```python
from build123d import *

# Parameters (mm, degrees)
SKETCH1_R           = 6.25
BOSS_EXTRUDE1_DEPTH = 20
BOSS_EXTRUDE2_DEPTH = 90
SKETCH3_R           = 1.75
CUT_EXTRUDE1_DEPTH  = 109.72585939
FILLET1_R           = 3
FILLET2_R           = 5


with BuildPart() as part:
    # Sketch1 → Boss-Extrude1 (new body)
    with BuildSketch(Plane(origin=(0, 0, 0), x_dir=(1, 0, 0), z_dir=(0, 1, 0))):
        with BuildLine():
            Line((0, 9.75), (11.25, 9.75))
            ThreePointArc((11.25, 9.75), (14.785533906, 8.285533906), (16.25, 4.75))
            Line((16.25, 4.75), (16.25, -9.75))
            Line((16.25, -9.75), (0, -9.75))
            ThreePointArc((0, -9.75), (-9.75, 0), (0, 9.75))
        make_face()
        with Locations(Location((0, 0, 0), (0, 0, 270))):
            Circle(SKETCH1_R, mode=Mode.SUBTRACT)
    extrude(amount=BOSS_EXTRUDE1_DEPTH)

    # Sketch2 → Boss-Extrude2 (add)
    with BuildSketch(Plane(origin=(16.25, 0, 0), x_dir=(0, 0, -1), z_dir=(1, 0, 0))):
        with BuildLine():
            Line((-6.75, 6), (-4.75, 6))
            ThreePointArc((-4.75, 6), (-2.628679656, 6.878679656), (-1.75, 9))
            Line((-1.75, 9), (-1.75, 11))
            ThreePointArc((-1.75, 11), (-2.628679656, 13.121320344), (-4.75, 14))
            Line((-4.75, 14), (-6.75, 14))
            ThreePointArc((-6.75, 14), (-8.871320344, 13.121320344), (-9.75, 11))
            Line((-9.75, 11), (-9.75, 9))
            ThreePointArc((-9.75, 9), (-8.871320344, 6.878679656), (-6.75, 6))
        make_face()
    extrude(amount=BOSS_EXTRUDE2_DEPTH)

    # Sketch3 → Cut-Extrude1 (cut, through all)
    with BuildSketch(Plane(origin=(0, 0, 1.75), x_dir=(-1, 0, 0), z_dir=(0, 0, -1))):
        with Locations(Location((-101.25, 10, 0), (0, 0, 34.849904579))):
            Circle(SKETCH3_R)
        with Locations(Location((-96.25, 10, 0), (0, 0, 34.849904579))):
            Circle(SKETCH3_R)
        with Locations(Location((-91.25, 10, 0), (0, 0, 34.849904579))):
            Circle(SKETCH3_R)
        with Locations(Location((-86.25, 10, 0), (0, 0, 34.849904579))):
            Circle(SKETCH3_R)
        with Locations(Location((-81.25, 10, 0), (0, 0, 34.849904579))):
            Circle(SKETCH3_R)
    extrude(amount=-CUT_EXTRUDE1_DEPTH, mode=Mode.SUBTRACT)

    # Fillet1
    fillet1_edges = [part.edges().sort_by_distance(p)[0] for p in [
        (106.25, 6.878679656, 8.871320344),
        (106.25, 6, 5.75),
        (106.25, 6.878679656, 2.628679656),
        (106.25, 10, 1.75),
        (106.25, 13.121320344, 2.628679656),
        (106.25, 14, 5.75),
        (106.25, 13.121320344, 8.871320344),
        (106.25, 10, 9.75),
    ]]
    fillet(fillet1_edges, radius=FILLET1_R)

    # Fillet2
    # the kernel refuses this fillet: 5 mm, written as the material it adds along each edge
    with BuildSketch(Plane(origin=(16.25, 9, 6.75), x_dir=(1.1842378929335002e-15, -0.8556201630305047, -0.5176042277799251), z_dir=(0, -0.5176042277799251, 0.8556201630305047))) as fillet2_piece_1_section:
        with BuildLine():
            CenterArc((-3 - FILLET2_R, FILLET2_R), FILLET2_R, 270, 90)
            Line((-3, FILLET2_R), (-3, 0))
            Line((-3, 0), (-3 - FILLET2_R, 0))
        make_face()
    fillet2_piece_1 = revolve(axis=Axis((16.25, 9, 6.75), (1, 0, 0)), revolution_arc=328.828315396, mode=Mode.PRIVATE)
    fillet2_piece_1 = split(fillet2_piece_1, bisect_by=Plane(origin=(16.92449451, 12.664519723, 9.75), z_dir=(0, 0, -1)), keep=Keep.TOP, mode=Mode.PRIVATE)
    add(fillet2_piece_1)
    with BuildSketch(Plane(origin=(16.25, 6, 6.75), x_dir=(0, -1, 0), z_dir=(0, 0, -1)), Plane(origin=(16.25, 9, 1.75), x_dir=(0, 0, -1), z_dir=(0, 1, 0))) as fillet2_piece_2:
        with BuildLine():
            CenterArc((FILLET2_R, -FILLET2_R), FILLET2_R, 90, 90)
            Line((0, -FILLET2_R), (0, 0))
            Line((0, 0), (FILLET2_R, 0))
        make_face()
    extrude(amount=2)
    with BuildSketch(Plane(origin=(16.25, 9, 4.75), x_dir=(0, -1, 0), z_dir=(0, 0, 1))) as fillet2_piece_3:
        with BuildLine():
            CenterArc((3 + FILLET2_R, FILLET2_R), FILLET2_R, 180, 90)
            Line((3, FILLET2_R), (3, 0))
            Line((3, 0), (3 + FILLET2_R, 0))
        make_face()
    revolve(axis=Axis((16.25, 9, 4.75), (1, 0, 0)), revolution_arc=90)
    with BuildSketch(Plane(origin=(16.25, 11, 4.75), x_dir=(0, 0, -1), z_dir=(0, -1, 0))) as fillet2_piece_4:
        with BuildLine():
            CenterArc((3 + FILLET2_R, FILLET2_R), FILLET2_R, 180, 90)
            Line((3, FILLET2_R), (3, 0))
            Line((3, 0), (3 + FILLET2_R, 0))
        make_face()
    revolve(axis=Axis((16.25, 11, 4.75), (1, 0, 0)), revolution_arc=90)
    with BuildSketch(Plane(origin=(16.25, 14, 4.75), x_dir=(1, 0, 0), z_dir=(0, 0, 1))) as fillet2_piece_5:
        with BuildLine():
            CenterArc((FILLET2_R, FILLET2_R), FILLET2_R, 180, 90)
            Line((0, FILLET2_R), (0, 0))
            Line((0, 0), (FILLET2_R, 0))
        make_face()
    extrude(amount=2)
    with BuildSketch(Plane(origin=(16.25, 11, 6.75), x_dir=(0, 1, 0), z_dir=(0, 0, -1))) as fillet2_piece_6_section:
        with BuildLine():
            CenterArc((3 + FILLET2_R, FILLET2_R), FILLET2_R, 180, 90)
            Line((3 + FILLET2_R, 0), (3, 0))
            Line((3, 0), (3, FILLET2_R))
        make_face()
    fillet2_piece_6 = revolve(axis=Axis((16.25, 11, 6.75), (1, 0, 0)), revolution_arc=328.828315396, mode=Mode.PRIVATE)
    fillet2_piece_6 = split(fillet2_piece_6, bisect_by=Plane(origin=(17.971658099, 13.274254424, 9.75), z_dir=(0, 0, -1)), keep=Keep.TOP, mode=Mode.PRIVATE)
    add(fillet2_piece_6)


solid = part.part
```
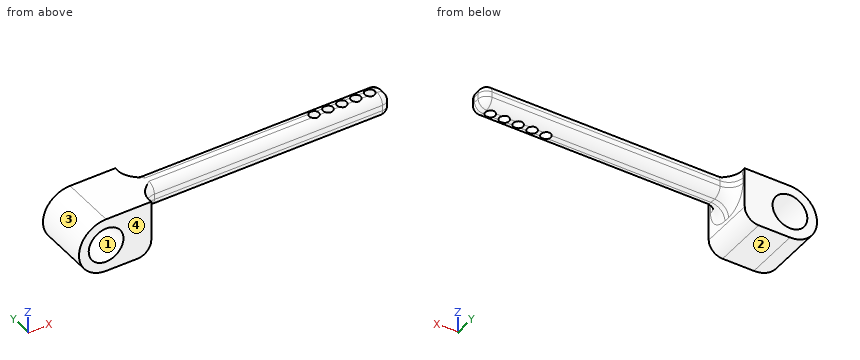
Can you work these out from the model? Positions are in its coordinate system, mm. Face numbers are marked on the shaded views. Give positions to 0.01 mm unless a question says otherwise; leave off trailing zeros. Loops run counter-clockwise (first coordinate to the right, second up) from the corner with the lowest first, then second, coordinate; pieces in that order, holes last. Notation, with made-up numbers: M 52,62.5 L 63,62.5 A11 ccw 63,76.5 Z; hole C 62.25,87.5 d2. An arc over 180 degrees is marked long. Answer in a Markdown table with one row per item.
1. If I drill on line 1 along Z through (x, y) = (-0.5, 7); line 2 along Y through (x, z) = (101.25, 4.5); line 3 along X through (y, z) = (3, -3.5), over which ranges is the centre line in solid material (lowest first)?
Taken from the geometry:
| item | result |
|---|---|
| line 1 | z = -9.74 to -6.23, 6.23 to 9.74 |
| line 2 | y = 6.01 to 8.25, 11.75 to 13.99 |
| line 3 | x = -9.1 to -5.18, 5.18 to 16.25 |
2. For pin 1 Ø2 at (y, z) = (6, 7) entering from -X; pin 2 Ø4 at (y, z) = (16, 4) entering from -X; pin 3 Ø2 at (x, y) = (94, 9.5) entering from -Z, each with a flat end and sliding along its axis, tell me the tip position at first contact or that it passes through.
Taken from the geometry:
| item | result |
|---|---|
| pin 1 | stops at x = -7.69 |
| pin 2 | stops at x = -9.54 |
| pin 3 | stops at z = 1.75 |
3. Suppose I cut it at A-A on x = 101.25. Write out the boundary of the cut face in (y, z).
Taken from the geometry:
| item | result |
|---|---|
| outline | M 6,4.75 A3 ccw 8.25,1.85 L 8.25,9.65 A3 ccw 6,6.75 Z; M 11.75,1.85 A3 ccw 14,4.75 L 14,6.75 A3 ccw 11.75,9.65 Z |
4. Thinking about a two-plate mould opening in Z: for the marked faces 1, 2, 3 and 4, which applies, released by +Z, released by -Z, zero draft, split by the parting line, or undercut?
Taken from the geometry:
| item | result |
|---|---|
| face 1 | undercut |
| face 2 | released by -Z |
| face 3 | split by the parting line |
| face 4 | zero draft |
